```python
from build123d import *

# Parameters (mm, degrees)
SKIZZE1_W                       = 45
SKIZZE1_H                       = 65
AUFSATZ_LINEAR_AUSTRAGEN1_DEPTH = 3
VERRUNDUNG1_R                   = 3
SKIZZE2_R                       = 1.75
SKIZZE2_R_2                     = 15
SCHNITT_LINEAR_AUSTRAGEN1_DEPTH = 12


with BuildPart() as part:
    # Skizze1 → Aufsatz-Linear austragen1 (new body)
    with BuildSketch(Plane.XY):
        Rectangle(SKIZZE1_W, SKIZZE1_H)
    extrude(amount=AUFSATZ_LINEAR_AUSTRAGEN1_DEPTH)

    # Verrundung1
    verrundung1_edges = [part.edges().sort_by_distance(p)[0] for p in [
        (-22.5, 32.5, 1.5),
        (22.5, 32.5, 1.5),
        (22.5, -32.5, 1.5),
        (-22.5, -32.5, 1.5),
    ]]
    fillet(verrundung1_edges, radius=VERRUNDUNG1_R)

    # Skizze2 → Schnitt-Linear austragen1 (cut)
    with BuildSketch(Plane.XY.offset(3)):
        with Locations((-15.5, -26.5)):
            Circle(SKIZZE2_R)
        with Locations((-15.5, 4.5)):
            Circle(SKIZZE2_R)
        with Locations((15.5, 4.5)):
            Circle(SKIZZE2_R)
        with Locations((15.5, -26.5)):
            Circle(SKIZZE2_R)
        with Locations((15.5, 22.5)):
            Circle(SKIZZE2_R)
        with Locations((-15.5, 22.5)):
            Circle(SKIZZE2_R)
        with Locations((0, -11)):
            Circle(SKIZZE2_R_2)
    extrude(amount=-SCHNITT_LINEAR_AUSTRAGEN1_DEPTH, mode=Mode.SUBTRACT)


solid = part.part
```
Verification items for the finished model (mm, model axes). Coordinates: 2 decimals unless noted, no trailing zeros. Order: outer loops, then holes, each group sorted by start corner. A loop starts at its lowest first (then second) coordinate and runs counter-clockwise, first axis right, second up. Notation, with made-up numbers: (62, -11) - (100, -11) arc R12 ccw to (100, 6) - close; hole circle Ø1 at (73, -32). An arc over 180 degrees is marked (long way). Return JSON: item names as keys, results as strings.
(1) Go/stop test with a flat-tipped pin: pin 1 (3 mm diameter, centred on x = -15.5, y = -26.5, fed in from -Z). Record where the tip stops, or that it passes through.
Filled sheet:
{"pin 1": "passes through"}
(2) Section check D-D, the plane y = 22.5. Record the cut outline in (x, z), and give its area (3 significant figures).
Filled sheet:
{"outline": "(-22.5, 0) - (-17.25, 0) - (-17.25, 3) - (-22.5, 3) - close; (-13.75, 0) - (13.75, 0) - (13.75, 3) - (-13.75, 3) - close; (17.25, 0) - (22.5, 0) - (22.5, 3) - (17.25, 3) - close", "area": "114 mm^2"}
(3) Section check C-C, the plane z = 0.55. Record the cut outline in (x, y), and give its area (3 significant figures).
Filled sheet:
{"outline": "(-22.5, -29.5) arc R3 ccw to (-19.5, -32.5) - (19.5, -32.5) arc R3 ccw to (22.5, -29.5) - (22.5, 29.5) arc R3 ccw to (19.5, 32.5) - (-19.5, 32.5) arc R3 ccw to (-22.5, 29.5) - close; hole circle Ø3.5 at (-15.5, -26.5); hole circle Ø3.5 at (-15.5, 4.5); hole circle Ø3.5 at (-15.5, 22.5); hole circle Ø30 at (0, -11); hole circle Ø3.5 at (15.5, -26.5); hole circle Ø3.5 at (15.5, 4.5); hole circle Ø3.5 at (15.5, 22.5)", "area": "2,150 mm^2"}
(4) Section check A-A, the plane x = 0. Record the cut outline in (y, z).
Filled sheet:
{"outline": "(-32.5, 0) - (-26, 0) - (-26, 3) - (-32.5, 3) - close; (4, 0) - (32.5, 0) - (32.5, 3) - (4, 3) - close"}
(5) Section check B-B, the plane y = -2. Record the cut outline in (x, z).
Filled sheet:
{"outline": "(-22.5, 0) - (-12, 0) - (-12, 3) - (-22.5, 3) - close; (12, 0) - (22.5, 0) - (22.5, 3) - (12, 3) - close"}
(6) Mould release check, pull along X, two halves, no side actions. Record for faces 1 (the cylindrical face through (21.64, 31.6, 1.52)), 2 (the flat face through (0, 8, 0)), 3 (the cylindrical face through (-15.728, -24.765, 1.521)), 4 (the cylindrical face through (-11.056, -0.862, 1.521)): pulls with the +X half, pulls with the -X half, needs draft (parallel to the pull), parting line crosses it, or undercut.
Filled sheet:
{"face 1": "pulls with the +X half", "face 2": "needs draft", "face 3": "undercut", "face 4": "undercut"}
(7) Thickness scan on line 1 along Y through (x, z) = (-15.5, 2.4); line 2 along Y through (x, z) = (17, 0.35); line 3 along Y through (x, z) = (0, 2.6). Record the ranges inside material, lowest first.
Filled sheet:
{"line 1": "y = -32.5 to -28.25, -24.75 to 2.75, 6.25 to 20.75, 24.25 to 32.5", "line 2": "y = -32.5 to -27.4, -25.6 to 3.6, 5.4 to 21.6, 23.4 to 32.5", "line 3": "y = -32.5 to -26, 4 to 32.5"}
